from build123d import *

# Parameters (mm, degrees)
F1_DEPTH = 25.4
F3_DEPTH = 25.4
F4_W     = 12.683143
F4_H     = 12.7472
F5_DEPTH = 25.4


with BuildPart() as f1:
    # F0 (on Right) → F1 (new body)
    with BuildSketch(Plane.YZ):
        Polygon((-20.469976, 32.562451), (-45.869976, 32.76404), (-45.869976, 1.01404), (-20.469976, 1.01404), align=None)
    extrude(amount=F1_DEPTH)

    # F2 (on face) → F3 (cut)
    with BuildSketch(Plane.YZ.offset(25.4)):
        Polygon((-20.469976, 32.562451), (-33.169976, 32.663246), (-20.469976, 13.71404), align=None)
    extrude(amount=-F3_DEPTH, mode=Mode.SUBTRACT)

    # F4 (on Right) → F5 (join)
    with BuildSketch(Plane.YZ):
        with Locations((-14.194957, 7.370238)):
            Rectangle(F4_W, F4_H)
    extrude(amount=F5_DEPTH)


solid = f1.part
Can you work these out from the model? Positions are in its coordinate system, mm. A direction names the side the tool comes from. Give positions to 0.01 mm unless a question says otherwise; leave off trailing zeros. Write each loop counter-clockwise with the first axis right and the second up, starting at its lowest first coordinate (ties: lowest second). Pieces come first, ordered by that corner, then holes. Notation, with made-up numbers: M 44.25,-25 L 56.25,-25 A9 ccw 56.25,-9 Z; hole C 25,1.25 d5. An arc over 180 degrees is marked long. Answer in a Markdown table with one row per item. Add a question column.
Item 1: On a 3-axis mill with a long thin cutter (end or side, diameter ignored), from which of +Z, -Z, +X, -X, +Y, -Y can I reach the whole of each face in a straight line? I mean faces 1 (the flat face through (13, -14, 13.744)), 2 (the flat face through (13, -7.853, 7)). Say none if no direction works.
Item 2: Please list where these lines run through material, in increasing order: L1, parallel to Z at x = 20.5, y = -33.5; L2, parallel to Z at x = 4.5, y = -20; L3, parallel to Y at x = 4, z = 25.
Item 3: Imagine slicing it at B-B, the plane y = -19.5. Write out the boundary of the cut face in (x, z).
Item 4: Imagine slicing it at C-C, the plane z = 26.5. Write out the boundary of the cut face in (x, y), plus the area to 4 significant figures.
Item 5: For pin 1 Ø12.5 at (x, y) = (18, -31.5) entering from -Z; pin 2 Ø6.5 at (x, y) = (7, -15) entering from +Z; pin 3 Ø12 at (x, y) = (7, -26.5) entering from +Z, each with a flat end and sliding along its axis, tell me the tip position at first contact or that it passes through.
Evaluation:
| question | item | result |
|---|---|---|
| 1 | face 1 | +Z, +X, -X, +Y |
| 1 | face 2 | +Z, -Z, +X, -X, +Y |
| 2 | L1 | z = 1.01 to 32.67 |
| 2 | L2 | z = 1 to 13.74 |
| 2 | L3 | y = -45.87 to -28.03 |
| 3 | outline | M 0,1 L 25.4,1 L 25.4,13.74 L 0,13.74 Z |
| 4 | outline | M 0,-45.87 L 25.4,-45.87 L 25.4,-29.04 L 0,-29.04 Z |
| 4 | area | 427.5 mm² |
| 5 | pin 1 | stops at z = 1.01 |
| 5 | pin 2 | stops at z = 13.74 |
| 5 | pin 3 | stops at z = 31.66 |
